from build123d import *

# Parameters (mm, degrees)
CYLINDER_R        = 2.55
CYLINDER_DEPTH    = 7.6
FILLET_R          = 2.5
PAD_DEPTH         = 5
CYLINDER001_R     = 3.75
CYLINDER001_DEPTH = 8.8
FILLET001_R       = 3.74
FILLET002_R       = 0.5


with BuildPart() as led_clearance_to_be_removed:
    # Cylinder → Cylinder (new body)
    with BuildSketch(Plane.XY.offset(-0.01)):
        Circle(CYLINDER_R)
    extrude(amount=CYLINDER_DEPTH)

    # Fillet
    fillet_edges = [led_clearance_to_be_removed.edges().sort_by_distance(p)[0] for p in [
        (-2.55, 0, 7.59),
    ]]
    fillet(fillet_edges, radius=FILLET_R)


with BuildPart() as flame_shape:
    # Sketch → Pad (new body)
    with BuildSketch(Plane.XZ):
        with BuildLine():
            Line((-4, 0), (4, 0))
            ThreePointArc((4, 0), (5.213606, 6.5), (4, 13))
            ThreePointArc((4, 25), (2.338096, 19), (4, 13))
            ThreePointArc((4, 25), (-3.734918, 13.695174), (-4, 0))
        make_face()
    extrude(amount=PAD_DEPTH)


with BuildPart() as flame_shape_1:
    # Body placement: moved
    add(flame_shape.part.moved(Location((0, 2.5, 0))))


with BuildPart() as flame_diffuser:
    # Cylinder001 → Cylinder001 (new body)
    with BuildSketch(Plane.XY):
        Circle(CYLINDER001_R)
    extrude(amount=CYLINDER001_DEPTH)

    # Fillet001
    fillet001_edges = [flame_diffuser.edges().sort_by_distance(p)[0] for p in [
        (-3.75, 0, 8.8),
    ]]
    fillet(fillet001_edges, radius=FILLET001_R)

    # Fusion: union flame shape
    add(flame_shape_1.part)

    # Cut: cut led clearance to be removed
    add(led_clearance_to_be_removed.part, mode=Mode.SUBTRACT)

    # Fillet002
    fillet002_edges = [flame_diffuser.edges().sort_by_distance(p)[0] for p in [
        (4, 0, 25),
    ]]
    fillet(fillet002_edges, radius=FILLET002_R)


solid = flame_diffuser.part
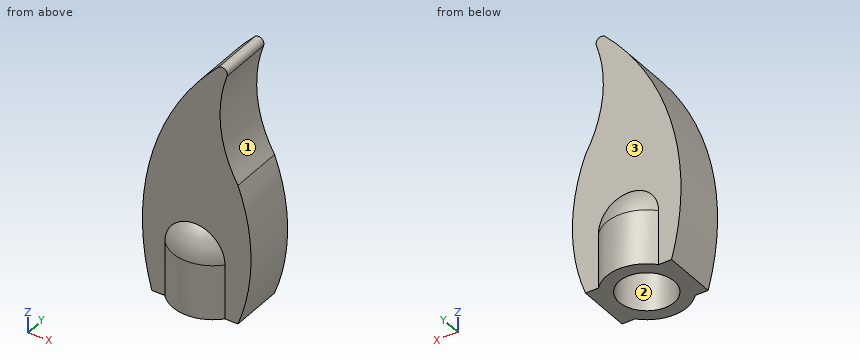
For this review, take the finished solid that the model builds, in its own axes (mm). Face numbers are marked on the shaded views. Coordinates: 2 decimals unless noted, no trailing zeros. Order: outer loops, then holes, each group sorted by start corner. A loop starts at its lowest first (then second) coordinate and runs counter-clockwise, first axis right, second up. Notation, with made-up numbers: (53, 14.25) - (72, 14.25) arc R28 ccw to (72, 44.25) - close; hole circle Ø9 at (89, 86.25). An arc over 180 degrees is marked (long way). Use one line per item in the form item = value.
Q1. Consider section B-B (x = 4.75). Give the boundary of the cut face in (y, z), then the cut area to 3 significant figures.
Checked values:
outline = (-2.5, 2.44) - (2.5, 2.44) - (2.5, 10.56) - (-2.5, 10.56) - close
area = 40.6 mm2
Q2. Draft analysis for pull direction Y (two halves, no side actions). For the marked faces 1, 2 and 3, state which applies: +Y half, -Y half, draft (parallel to the pull), parting line (faces both ways), or undercut.
Checked values:
face_1 = draft
face_2 = undercut
face_3 = +Y half
Q3. Consider section C-C (z = 21.5). Give the boundary of the cut face in (x, y).
Checked values:
outline = (0.49, -2.5) - (2.61, -2.5) - (2.61, 2.5) - (0.49, 2.5) - close
Q4. Consider section A-A (z = 3.25). Give the boundary of the cut face in (x, y).
Checked values:
outline = (-4.66, -2.5) - (-2.8, -2.5) arc R3.75 ccw to (2.8, -2.5) - (4.92, -2.5) - (4.92, 2.5) - (2.8, 2.5) arc R3.75 ccw to (-2.8, 2.5) - (-4.66, 2.5) - close; hole circle Ø5.1 at (0, 0)
Q5. For P1, Ø1, axis at x = -0.5, z = 19, coming from the +Y side; P2, Ø1.5, axis at y = 2.5, z = 16.5, coming from the +X side; P3, Ø2, axis at y = 1, z = 4, coming from the -X side, all flat-tipped, find the tip position at first contact; note any pin that passes through.
Checked values:
P1 = 2.5
P2 = 2.8
P3 = -4.83
Q6. For probe 1 along Y at (x, z) = (0, 3.55); probe 2 along Y at (x, z) = (0.75, 19); probe 3 along X at (y, z) = (2, 5.5), list the stretches that pass through material, from the lowest coordinate up. Write a range as from..to.
Checked values:
probe_1 = -3.75..-2.55, 2.55..3.75
probe_2 = -2.5..2.5
probe_3 = -4.86..-1.53, 1.53..5.19
